from build123d import *

# Parameters (mm, degrees)
BOSS_EXTRUDE2_DEPTH = 80
CUT_EXTRUDE3_DEPTH  = 88.451415083
SKETCH6_RX          = 8
SKETCH6_RY          = 4
CUT_EXTRUDE4_DEPTH  = 75
SKETCH7_R           = 1.5
CUT_EXTRUDE5_DEPTH  = 83.902050638


# Read off the part's stored shape, not the designer's step: Boss-Extrude2
with BuildPart() as part:
    # Boss-Extrude2 outline → Boss-Extrude2 (new body)
    with BuildSketch(Plane(origin=(0, 0, 0), x_dir=(1, 0, 0), z_dir=(0, 1, 0))):
        with BuildLine():
            Line((1.5, 24.954959427), (0.75, 20))
            Line((0.75, 20), (-0.75, 20))
            Line((-0.75, 20), (-1.5, 24.954959427))
            ThreePointArc((-1.5, 24.954959427), (-2.306708986, 24.893354407), (-3.111002112, 24.805678097))
            Line((-3.111002112, 24.805678097), (-2.937760532, 19.797274132))
            Line((-2.937760532, 19.797274132), (-4.412220181, 19.521649855))
            Line((-4.412220181, 19.521649855), (-6.059921411, 24.254429544))
            ThreePointArc((-6.059921411, 24.254429544), (-6.841574752, 24.045641079), (-7.616062779, 23.811669151))
            Line((-7.616062779, 23.811669151), (-6.525479152, 18.920375838))
            Line((-6.525479152, 18.920375838), (-7.924187496, 18.378513338))
            Line((-7.924187496, 18.378513338), (-10.413479467, 22.727944152))
            ThreePointArc((-10.413479467, 22.727944152), (-11.143458894, 22.379082284), (-11.861767562, 22.006782371))
            Line((-11.861767562, 22.006782371), (-9.890980406, 17.399166837))
            Line((-9.890980406, 17.399166837), (-11.166306109, 16.609518592))
            Line((-11.166306109, 16.609518592), (-14.412418969, 20.427485882))
            ThreePointArc((-14.412418969, 20.427485882), (-15.065865909, 19.950430682), (-15.703534077, 19.452481011))
            Line((-15.703534077, 19.452481011), (-12.919656185, 15.285450077))
            Line((-12.919656185, 15.285450077), (-14.028169561, 14.274906612))
            Line((-14.028169561, 14.274906612), (-17.920560829, 17.43139408))
            ThreePointArc((-17.920560829, 17.43139408), (-18.475222931, 16.842391091), (-19.010535574, 16.235748741))
            Line((-19.010535574, 16.235748741), (-15.508368568, 12.651205648))
            Line((-15.508368568, 12.651205648), (-16.412320523, 11.454179807))
            Line((-16.412320523, 11.454179807), (-20.818439483, 13.841697059))
            ThreePointArc((-20.818439483, 13.841697059), (-21.255428393, 13.160804072), (-21.670156083, 12.46612752))
            Line((-21.670156083, 12.46612752), (-17.56896206, 9.586139584))
            Line((-17.56896206, 9.586139584), (-18.237569594, 8.243394647))
            Line((-18.237569594, 8.243394647), (-23.00737115, 9.780637646))
            ThreePointArc((-23.00737115, 9.780637646), (-23.311805735, 9.031041655), (-23.591825416, 8.271987279))
            Line((-23.591825416, 8.271987279), (-19.031265621, 6.194629034))
            Line((-19.031265621, 6.194629034), (-19.441760106, 4.751890569))
            Line((-19.441760106, 4.751890569), (-24.412814386, 5.386510349))
            ThreePointArc((-24.412814386, 5.386510349), (-24.574327492, 4.593737945), (-24.71010343, 3.796154431))
            Line((-24.71010343, 3.796154431), (-19.845482256, 2.592167821))
            Line((-19.845482256, 2.592167821), (-19.983884795, 1.098566557))
            Line((-19.983884795, 1.098566557), (-24.986908509, 0.808951902))
            ThreePointArc((-24.986908509, 0.808951902), (-25, 0), (-24.986908509, -0.808951902))
            Line((-24.986908509, -0.808951902), (-19.983884795, -1.098566557))
            Line((-19.983884795, -1.098566557), (-19.845482256, -2.592167821))
            Line((-19.845482256, -2.592167821), (-24.71010343, -3.796154431))
            ThreePointArc((-24.71010343, -3.796154431), (-24.574327492, -4.593737945), (-24.412814386, -5.386510349))
            Line((-24.412814386, -5.386510349), (-19.441760106, -4.751890569))
            Line((-19.441760106, -4.751890569), (-19.031265621, -6.194629034))
            Line((-19.031265621, -6.194629034), (-23.591825416, -8.271987279))
            ThreePointArc((-23.591825416, -8.271987279), (-23.311805735, -9.031041655), (-23.00737115, -9.780637646))
            Line((-23.00737115, -9.780637646), (-18.237569594, -8.243394647))
            Line((-18.237569594, -8.243394647), (-17.56896206, -9.586139584))
            Line((-17.56896206, -9.586139584), (-21.670156083, -12.46612752))
            ThreePointArc((-21.670156083, -12.46612752), (-21.255428393, -13.160804072), (-20.818439483, -13.841697059))
            Line((-20.818439483, -13.841697059), (-16.412320523, -11.454179807))
            Line((-16.412320523, -11.454179807), (-15.508368568, -12.651205648))
            Line((-15.508368568, -12.651205648), (-19.010535574, -16.235748741))
            ThreePointArc((-19.010535574, -16.235748741), (-18.475222931, -16.842391091), (-17.920560829, -17.43139408))
            Line((-17.920560829, -17.43139408), (-14.028169561, -14.274906612))
            Line((-14.028169561, -14.274906612), (-12.919656185, -15.285450077))
            Line((-12.919656185, -15.285450077), (-15.703534077, -19.452481011))
            ThreePointArc((-15.703534077, -19.452481011), (-15.065865909, -19.950430682), (-14.412418969, -20.427485882))
            Line((-14.412418969, -20.427485882), (-11.166306109, -16.609518592))
            Line((-11.166306109, -16.609518592), (-9.890980406, -17.399166837))
            Line((-9.890980406, -17.399166837), (-11.861767562, -22.006782371))
            ThreePointArc((-11.861767562, -22.006782371), (-11.143458894, -22.379082284), (-10.413479467, -22.727944152))
            Line((-10.413479467, -22.727944152), (-7.924187496, -18.378513338))
            Line((-7.924187496, -18.378513338), (-6.525479152, -18.920375838))
            Line((-6.525479152, -18.920375838), (-7.616062779, -23.811669151))
            ThreePointArc((-7.616062779, -23.811669151), (-6.841574752, -24.045641079), (-6.059921411, -24.254429544))
            Line((-6.059921411, -24.254429544), (-4.412220181, -19.521649855))
            Line((-4.412220181, -19.521649855), (-2.937760532, -19.797274132))
            Line((-2.937760532, -19.797274132), (-3.111002112, -24.805678097))
            ThreePointArc((-3.111002112, -24.805678097), (-2.306708986, -24.893354407), (-1.5, -24.954959427))
            Line((-1.5, -24.954959427), (-0.75, -20))
            Line((-0.75, -20), (0.75, -20))
            Line((0.75, -20), (1.5, -24.954959427))
            ThreePointArc((1.5, -24.954959427), (2.306708986, -24.893354407), (3.111002112, -24.805678097))
            Line((3.111002112, -24.805678097), (2.937760532, -19.797274132))
            Line((2.937760532, -19.797274132), (4.412220181, -19.521649855))
            Line((4.412220181, -19.521649855), (6.059921411, -24.254429544))
            ThreePointArc((6.059921411, -24.254429544), (6.841574752, -24.045641079), (7.616062779, -23.811669151))
            Line((7.616062779, -23.811669151), (6.525479152, -18.920375838))
            Line((6.525479152, -18.920375838), (7.924187496, -18.378513338))
            Line((7.924187496, -18.378513338), (10.413479467, -22.727944152))
            ThreePointArc((10.413479467, -22.727944152), (11.143458894, -22.379082284), (11.861767562, -22.006782371))
            Line((11.861767562, -22.006782371), (9.890980406, -17.399166837))
            Line((9.890980406, -17.399166837), (11.166306109, -16.609518592))
            Line((11.166306109, -16.609518592), (14.412418969, -20.427485882))
            ThreePointArc((14.412418969, -20.427485882), (15.065865909, -19.950430682), (15.703534077, -19.452481011))
            Line((15.703534077, -19.452481011), (12.919656185, -15.285450077))
            Line((12.919656185, -15.285450077), (14.028169561, -14.274906612))
            Line((14.028169561, -14.274906612), (17.920560829, -17.43139408))
            ThreePointArc((17.920560829, -17.43139408), (18.475222931, -16.842391091), (19.010535574, -16.235748741))
            Line((19.010535574, -16.235748741), (15.508368568, -12.651205648))
            Line((15.508368568, -12.651205648), (16.412320523, -11.454179807))
            Line((16.412320523, -11.454179807), (20.818439483, -13.841697059))
            ThreePointArc((20.818439483, -13.841697059), (21.255428393, -13.160804072), (21.670156083, -12.46612752))
            Line((21.670156083, -12.46612752), (17.56896206, -9.586139584))
            Line((17.56896206, -9.586139584), (18.237569594, -8.243394647))
            Line((18.237569594, -8.243394647), (23.00737115, -9.780637646))
            ThreePointArc((23.00737115, -9.780637646), (23.311805735, -9.031041655), (23.591825416, -8.271987279))
            Line((23.591825416, -8.271987279), (19.031265621, -6.194629034))
            Line((19.031265621, -6.194629034), (19.441760106, -4.751890569))
            Line((19.441760106, -4.751890569), (24.412814386, -5.386510349))
            ThreePointArc((24.412814386, -5.386510349), (24.574327492, -4.593737945), (24.71010343, -3.796154431))
            Line((24.71010343, -3.796154431), (19.845482256, -2.592167821))
            Line((19.845482256, -2.592167821), (19.983884796, -1.098566557))
            Line((19.983884796, -1.098566557), (24.986908509, -0.808951902))
            ThreePointArc((24.986908509, -0.808951902), (25, 0), (24.986908509, 0.808951902))
            Line((24.986908509, 0.808951902), (19.983884796, 1.098566557))
            Line((19.983884796, 1.098566557), (19.845482256, 2.592167821))
            Line((19.845482256, 2.592167821), (24.71010343, 3.796154431))
            ThreePointArc((24.71010343, 3.796154431), (24.574327492, 4.593737945), (24.412814386, 5.386510349))
            Line((24.412814386, 5.386510349), (19.441760106, 4.751890569))
            Line((19.441760106, 4.751890569), (19.031265621, 6.194629034))
            Line((19.031265621, 6.194629034), (23.591825416, 8.271987279))
            ThreePointArc((23.591825416, 8.271987279), (23.311805735, 9.031041655), (23.00737115, 9.780637646))
            Line((23.00737115, 9.780637646), (18.237569594, 8.243394647))
            Line((18.237569594, 8.243394647), (17.56896206, 9.586139584))
            Line((17.56896206, 9.586139584), (21.670156083, 12.46612752))
            ThreePointArc((21.670156083, 12.46612752), (21.255428393, 13.160804072), (20.818439483, 13.841697059))
            Line((20.818439483, 13.841697059), (16.412320523, 11.454179807))
            Line((16.412320523, 11.454179807), (15.508368568, 12.651205648))
            Line((15.508368568, 12.651205648), (19.010535574, 16.235748741))
            ThreePointArc((19.010535574, 16.235748741), (18.475222931, 16.842391091), (17.920560829, 17.43139408))
            Line((17.920560829, 17.43139408), (14.028169561, 14.274906612))
            Line((14.028169561, 14.274906612), (12.919656185, 15.285450077))
            Line((12.919656185, 15.285450077), (15.703534077, 19.452481011))
            ThreePointArc((15.703534077, 19.452481011), (15.065865909, 19.950430682), (14.412418969, 20.427485882))
            Line((14.412418969, 20.427485882), (11.166306109, 16.609518592))
            Line((11.166306109, 16.609518592), (9.890980406, 17.399166837))
            Line((9.890980406, 17.399166837), (11.861767562, 22.006782371))
            ThreePointArc((11.861767562, 22.006782371), (11.143458894, 22.379082284), (10.413479467, 22.727944152))
            Line((10.413479467, 22.727944152), (7.924187496, 18.378513338))
            Line((7.924187496, 18.378513338), (6.525479152, 18.920375838))
            Line((6.525479152, 18.920375838), (7.616062779, 23.811669151))
            ThreePointArc((7.616062779, 23.811669151), (6.841574752, 24.045641079), (6.059921411, 24.254429544))
            Line((6.059921411, 24.254429544), (4.412220181, 19.521649855))
            Line((4.412220181, 19.521649855), (2.937760532, 19.797274132))
            Line((2.937760532, 19.797274132), (3.111002112, 24.805678097))
            ThreePointArc((3.111002112, 24.805678097), (2.306708986, 24.893354407), (1.5, 24.954959427))
        make_face()
    extrude(amount=BOSS_EXTRUDE2_DEPTH)

    # Sketch5 → Cut-Extrude3 (cut, through all)
    with BuildSketch(Plane.XZ):
        with BuildLine():
            Line((-12.5, 6.623664739), (12.5, 6.623664739))
            ThreePointArc((12.5, 6.623664739), (0, 15.524722913), (-12.5, 6.623664739))
        make_face()
        with BuildLine():
            Line((12.5, -6.623664739), (-12.5, -6.623664739))
            ThreePointArc((-12.5, -6.623664739), (0, -15.524722913), (12.5, -6.623664739))
        make_face()
    extrude(amount=-CUT_EXTRUDE3_DEPTH, mode=Mode.SUBTRACT)

    # Sketch6 → Cut-Extrude4 (cut)
    with BuildSketch(Plane(origin=(0, 0, 0), x_dir=(-1, 0, 0), z_dir=(0, -1, 0))):
        with Locations((0, 0)):
            Ellipse(SKETCH6_RX, SKETCH6_RY)
    extrude(amount=-CUT_EXTRUDE4_DEPTH, mode=Mode.SUBTRACT)

    # Sketch7 → Cut-Extrude5 (cut, through all)
    with BuildSketch(Plane.XZ.offset(-75)):
        with Locations(Location((0, 0, 0), (0, 0, 270))):
            Circle(SKETCH7_R)
    extrude(amount=-CUT_EXTRUDE5_DEPTH, mode=Mode.SUBTRACT)


solid = part.part
Model file for the job. Use its own axes, mm. A direction names the side the tool comes from. Coordinates: 2 decimals unless noted, no trailing zeros. Return JSON: item names as keys, results as strings.
1. Flat gauge pins, fed straight in: pin 1 (10 mm diameter, centred on y = 33, z = 18.5, fed in from -X); pin 2 (0.8 mm diameter, centred on x = 0, y = 21.5, fed in from -Z); pin 3 (8 mm diameter, centred on x = -17.5, y = 59.5, fed in from +Z). Where does each tip first touch, or does it go through?
Ans:
{"pin 1": "x = -21.04", "pin 2": "z = -20", "pin 3": "z = 20.43"}
2. Tool access for faces 1 (the face through (-1.12, 39.44, -22.44)), 2 (the face through (-21.962, 39.44, 5.074)): list every direction of +Z, -Z, +X, -X, +Y, -Y with a clear straight run to the whole face (end or side of a thin tool).
Ans:
{"face 1": "-Z, +Y, -Y", "face 2": "+Y, -Y"}
3. Drill centre lines: probe 1 along Z at (x, y) = (0, 16); probe 2 along X at (y, z) = (77.9, 0); probe 3 along Z at (x, y) = (22, 10.5). Where is each one in solid material? Low to high.
Ans:
{"probe 1": "-20 to -15.52, -6.62 to -4, 4 to 6.62, 15.52 to 20", "probe 2": "-25 to -1.5, 1.5 to 25", "probe 3": "-9.46 to -7.55, -5.08 to -3.13, -0.98 to 0.98, 3.13 to 5.08, 7.55 to 9.46"}
4. Pull direction X, two halves, no side cores. Call faces 3 (the face through (2.295, 39.44, 24.894)), 4 (the face through (7.063, 39.44, -21.332)), 5 (the face through (-22.3, 39.4, -3.2)), 6 (the face through (-14.33, 39.44, -17.4)): +X half, -X half, draft (parallel to the pull), parting line (faces both ways), or undercut.
Ans:
{"face 3": "+X half", "face 4": "undercut", "face 5": "-X half", "face 6": "undercut"}
5. Saw through at A-A (y = 72.5). Give the number of separate pieces and of enclosed holes in the cut face, and give its area (3 significant figures).
Ans:
{"separate pieces": "1", "enclosed holes": "3", "area": "1,160 mm^2"}
